Could you check a few things on this model? Use its own coordinates, in mm. A direction names the side the tool comes from. Round coordinates to 2 decimals unless told otherwise and drop trailing zeros. Loops run counter-clockwise (first coordinate to the right, second up) from the corner with the lowest first, then second, coordinate; pieces in that order, holes last.
from build123d import *

# Parameters (mm, degrees)
PAD014_DEPTH            = 350
FILLET013_R             = 150
FILLET014_R             = 15
PAD015_DEPTH            = 30
FILLET015_R             = 10
BODY010_PLACEMENT_ANGLE = 270


with BuildPart() as part:
    # Sketch194 → Pad014 (new body)
    with BuildSketch(Plane.XY):
        with BuildLine():
            Line((0, 350), (0, 0))
            Line((0, 0), (350, 0))
            Line((350, 0), (350, 350))
            ThreePointArc((350, 350), (175, 525), (0, 350))
        make_face()
    extrude(amount=PAD014_DEPTH)

    # Fillet013
    fillet013_edges = [part.edges().sort_by_distance(p)[0] for p in [
        (350, 175, 0),
        (175, 525, 0),
        (0, 175, 0),
    ]]
    fillet(fillet013_edges, radius=FILLET013_R)

    # Fillet014
    fillet014_edges = [part.edges().sort_by_distance(p)[0] for p in [
        (0, 175, 350),
        (175, 0, 350),
        (350, 175, 350),
        (175, 525, 350),
    ]]
    fillet(fillet014_edges, radius=FILLET014_R)

    # Sketch195 (on Face4 of Fillet013) → Pad015 (join)
    with BuildSketch(Plane.XY.offset(350)):
        with BuildLine():
            Line((-5, 85), (355, 85))
            Line((355, 85), (355, 345))
            ThreePointArc((355, 345), (175, 525), (-5, 345))
            Line((-5, 85), (-5, 345))
        make_face()
    extrude(amount=PAD015_DEPTH)

    # Fillet015
    fillet015_edges = [part.edges().sort_by_distance(p)[0] for p in [
        (355, 345, 365),
        (-5, 345, 365),
        (175, 525, 350),
        (175, 525, 380),
        (-5, 85, 365),
        (-5, 215, 350),
        (-5, 215, 380),
        (355, 85, 365),
        (355, 215, 350),
        (355, 215, 380),
    ]]
    fillet(fillet015_edges, radius=FILLET015_R)


with BuildPart() as part_1:
    # Body010 placement: moved
    add(part.part.moved(Location((1727, 3999, 0))).rotate(Axis((1727, 3999, 0), (0, 0, 1)), BODY010_PLACEMENT_ANGLE))


solid = part_1.part
Item 1: Will these pins go through, and if not, where does the flat tip stop? pin 1 (10 mm diameter, centred on y = 3886, z = 299, fed in from +X); pin 2 (1.5 mm diameter, centred on x = 2060.5, z = 213.5, fed in from -Y); pin 3 (9 mm diameter, centred on y = 3807.5, z = 358, fed in from -X).
Results list:
pin 1: stops at x = 2242.46
pin 2: stops at y = 3649
pin 3: stops at x = 1812
Item 2: If we section it at B-B, the plane z = 257.5: Please give me the cut outline in (x, y), then the cut area to 3 significant figures.
Results list:
outline: (1727, 3649) - (2077, 3649) arc R175 ccw to (2077, 3999) - (1727, 3999) - close
area: 171,000 mm2
Item 3: For faces 1 (the cylindrical face through (2251.958, 3820.152, 241.205)), 2 (the flat face through (1904, 3999, 241)), 3 (the flat face through (1777, 3826, 350)), 4 (the flat face through (1900, 3649, 241)), which set-ups out of +Z, -Z, +X, -X, +Y, -Y let a thin tool reach every point of the face, with its end or its side?
Results list:
face 1: -Z, +X
face 2: -Z, +X, -X, +Y
face 3: +Z, -X, +Y, -Y
face 4: -Z, +X, -X, -Y
Item 4: If I drill on line 1 along Y through (x, z) = (2057, 193); line 2 along Z through (x, y) = (2080, 3851); line 3 along X through (y, z) = (3965, 266), over which ranges is the centre line in solid material (lowest first)?
Results list:
line 1: y = 3649 to 3999
line 2: z = 0.02 to 380
line 3: x = 1727 to 2180.65
Item 5: If we section it at A-A, the plane x = 1974: Please give me the cut outline in (y, z), then the cut area to 3 significant figures.
Results list:
outline: (3644, 360) arc R10 ccw to (3654, 350) - (3664, 350) arc R15 ccw to (3649, 335) - (3649, 150) arc R150 ccw to (3799, 0) - (3849, 0) arc R150 ccw to (3999, 150) - (3999, 335) arc R15 ccw to (3984, 350) - (3994, 350) arc R10 ccw to (4004, 360) - (4004, 370) arc R10 ccw to (3994, 380) - (3654, 380) arc R10 ccw to (3644, 370) - close
area: 123,000 mm2
